from build123d import *

# Parameters (mm, degrees)
SKETCH1_R           = 7.5
SKETCH1_R_2         = 1.45
SKETCH1_R_3         = 1.5
SKETCH1_R_4         = 3.75
BOSS_EXTRUDE1_DEPTH = 1.5
FILLET1_R           = 10
CUT_EXTRUDE1_DEPTH  = 3


with BuildPart() as part:
    # Sketch1 → Boss-Extrude1 (new body, symmetric)
    with BuildSketch(Plane(origin=(0, 0, 0), x_dir=(0, 0, -1), z_dir=(1, 0, 0))):
        with BuildLine():
            Line((18.291561976, -12.5), (40, -7.5))
            ThreePointArc((40, -7.5), (32.5, 0), (40, 7.5))
            Line((40, 7.5), (20, 7.5))
            Line((20, 7.5), (8.291561976, 12.5))
            ThreePointArc((8.291561976, 12.5), (13.216910184, 7.093185827), (15, 0))
            ThreePointArc((15, 0), (13.216910184, -7.093185827), (8.291561976, -12.5))
            Line((8.291561976, -12.5), (18.291561976, -12.5))
        make_face()
        with Locations((40, 0)):
            Circle(SKETCH1_R)
        with Locations((40, 0)):
            Circle(SKETCH1_R_2, mode=Mode.SUBTRACT)
        with BuildLine():
            ThreePointArc((8.291561976, 12.5), (-15, 0), (8.291561976, -12.5))
            ThreePointArc((8.291561976, -12.5), (13.216910184, -7.093185827), (15, 0))
            ThreePointArc((15, 0), (13.216910184, 7.093185827), (8.291561976, 12.5))
        make_face()
        with Locations((0, -7)):
            Circle(SKETCH1_R_3, mode=Mode.SUBTRACT)
        with Locations((-7, 0)):
            Circle(SKETCH1_R_3, mode=Mode.SUBTRACT)
        Circle(SKETCH1_R_4, mode=Mode.SUBTRACT)
        with Locations((0, 7)):
            Circle(SKETCH1_R_3, mode=Mode.SUBTRACT)
        with Locations((7, 0)):
            Circle(SKETCH1_R_3, mode=Mode.SUBTRACT)
    extrude(amount=BOSS_EXTRUDE1_DEPTH, both=True)

    # Fillet1
    fillet1_edges = [part.edges().sort_by_distance(p)[0] for p in [
        (0, -12.5, -18.291561976),
        (0, -12.5, -8.291561976),
        (0, 12.5, -8.291561976),
        (0, 7.5, -20),
        (0, -7.5, -40),
    ]]
    fillet(fillet1_edges, radius=FILLET1_R)

    # Sketch2 → Cut-Extrude1 (cut)
    with BuildSketch(Plane(origin=(1.5, 0, 0), x_dir=(0, 0, -1), z_dir=(1, 0, 0))):
        Polygon((17, 1), (30, 1), (32, -1), (32, -3), (30, -5), (17, -5), (15, -3), (15, -1), align=None)
    extrude(amount=-CUT_EXTRUDE1_DEPTH, mode=Mode.SUBTRACT)


solid = part.part
Verification items for the finished model (mm, model axes). A direction names the side the tool comes from. Coordinates: 2 decimals unless noted, no trailing zeros. Order: outer loops, then holes, each group sorted by start corner. A loop starts at its lowest first (then second) coordinate and runs counter-clockwise, first axis right, second up. Notation, with made-up numbers: M -40,19 L -28,19 A29 ccw -28,55 Z; hole C 36.5,-19.5 d1. An arc over 180 degrees is marked long. One line per item, written item: value. Start each with the question number.
Item 1: Depth check by flat-ended pin: P1, Ø1, axis at x = -1, y = -8, coming from the +Z side; P2, Ø0.9, axis at x = 0.5, z = -25.5, coming from the +Y side; P3, Ø0.9, axis at x = 0.5, z = -22, coming from the -Y side. Enter the tip coordinate at first touch or a pass-through.
Item 2: Sectioned sample at B-B on x = 0.9. Record the cut outline in (y, z), then the cut area to 3 significant figures.
Item 3: Sectioned sample at C-C on z = 0. Record the cut outline in (x, y), then the cut area to 3 significant figures.
Item 4: Sectioned sample at A-A on y = 0. Record the cut outline in (x, z), then the cut area to 3 significant figures.
Item 5: Mould release check, pull along Z, two halves, no side actions. Record for faces 3 (the flat face through (0, 7.5, -31)), 4 (the cylindrical face through (-0.02, 12.49, -8.38)), 5 (the flat face through (0, 0, -31)), 6 (the cylindrical face through (-0.02, 0.06, -38.55)): pulls with the +Z half, pulls with the -Z half, needs draft (parallel to the pull), parting line crosses it, or undercut.
Item 6: Sectioned sample at D-D on z = -25. Record the cut outline in (x, y).
Item 7: Thickness scan on probe 1 along Y at (x, z) = (-0.5, 0); probe 2 along Z at (x, y) = (0.85, -2); probe 3 along Y at (x, z) = (-0.6, -1). Record the ranges inside material, lowest first.
Item 8: Access from +Z, -Z, +X, -X, +Y, -Y to the whole of each face (thin tool, end or side, straight path). Record for faces 1 (the cylindrical face through (0.02, 7.71, -20.01)), 2 (the flat face through (0, 0, -16)).
Calculated:
1. P1: z = 12.99
1. P2: y = 7.5
1. P3: y = -11.75
2. outline: M -13.5,-6.54 A10 cw -12.5,-10.9 L -12.5,-17.15 A10 ccw -12.24,-19.4 L -7.7,-39.13 A10 cw -7.48,-40.59 A7.5 ccw 7.5,-40 L 7.5,-22.05 A10 cw 8.3,-18.12 L 12.19,-9.02 A10 cw 12.83,-7.77 A15 ccw long Z; hole C -7,0 d3; hole M -5,-30 L -3,-32 L -1,-32 L 1,-30 L 1,-17 L -1,-15 L -3,-15 L -5,-17 Z; hole C 0,0 d7.5; hole C 0,-7 d3; hole C 0,7 d3; hole C 0,-40 d2.9; hole C 7,0 d3
2. area: 1,110 mm^2
3. outline: M -1.5,-15 L 1.5,-15 L 1.5,-8.5 L -1.5,-8.5 Z; M -1.5,-5.5 L 1.5,-5.5 L 1.5,-3.75 L -1.5,-3.75 Z; M -1.5,3.75 L 1.5,3.75 L 1.5,5.5 L -1.5,5.5 Z; M -1.5,8.5 L 1.5,8.5 L 1.5,15 L -1.5,15 Z
3. area: 49.5 mm^2
4. outline: M -1.5,-47.5 L 1.5,-47.5 L 1.5,-41.45 L -1.5,-41.45 Z; M -1.5,-38.55 L 1.5,-38.55 L 1.5,-31 L -1.5,-31 Z; M -1.5,-16 L 1.5,-16 L 1.5,-8.5 L -1.5,-8.5 Z; M -1.5,-5.5 L 1.5,-5.5 L 1.5,-3.75 L -1.5,-3.75 Z; M -1.5,3.75 L 1.5,3.75 L 1.5,5.5 L -1.5,5.5 Z; M -1.5,8.5 L 1.5,8.5 L 1.5,15 L -1.5,15 Z
4. area: 93.3 mm^2
5. face 3: needs draft
5. face 4: pulls with the -Z half
5. face 5: undercut
5. face 6: undercut
6. outline: M -1.5,-10.95 L 1.5,-10.95 L 1.5,-5 L -1.5,-5 Z; M -1.5,1 L 1.5,1 L 1.5,7.5 L -1.5,7.5 Z
7. probe 1: -15 to -8.5, -5.5 to -3.75, 3.75 to 5.5, 8.5 to 15
7. probe 2: -47.23 to -32, -15 to -3.17, 3.17 to 14.87
7. probe 3: -14.97 to -8.12, -5.88 to -3.61, 3.61 to 5.88, 8.12 to 14.97
8. face 1: -Z, +X, -X, +Y
8. face 2: +X, -X
